The listing builds one solid part. Answer for the finished solid, in the listing's coordinates (mm). Face numbers are marked on the shaded views. A direction names the side the tool comes from. Give positions to 0.01 mm unless a question says otherwise; leave off trailing zeros. Write each loop counter-clockwise with the first axis right and the second up, starting at its lowest first coordinate (ties: lowest second). Pieces come first, ordered by that corner, then holes. Notation, with made-up numbers: (58, 22.25) -> (73, 22.25) arc R26 ccw to (73, 40.25) -> close; hole circle Ø8 at (-31, 70.25). An arc over 180 degrees is marked (long way). Put each result on its own line as item: value. Start each with the question number.
1) A cutting plane is placed at A-A (z = 0). Write down the section's boundary in (x, y), then the cut area to 4 significant figures.
2) For the marked faces 4 and 5, determine the directions among +Z, -Z, +X, -X, +Y, -Y from which every point of the face is accessible in a straight line to the end or side of a thin tool.
3) A cutting plane is placed at D-D (x = 2). Write down the section's boundary in (y, z), then the cut area to 3 significant figures.
4) Flat-ended cylindrical pins translate along their axes: pin 1 Ø1 at (x, z) = (1, 0.5) entering from +Y; pin 2 Ø2 at (x, z) = (-1, -1) entering from +Y. Find the tip coordinate at first contact, or state that the pin passes through.
5) A cutting plane is placed at B-B (x = 0). Write down the section's boundary in (y, z).
6) Find the intervals of material crossed by line 1 along X through (y, z) = (3, 0); line 2 along X through (y, z) = (7.2, 0), in increasing order. Write a range as from..to.
7) A cutting plane is placed at C-C (y = 5). Write down the section's boundary in (x, z).
8) For a pull along X with two mould halves and no side action, classify the marked faces 1, 2 and 3 as released by +X, released by -X, zero draft, split by the parting line, or undercut.
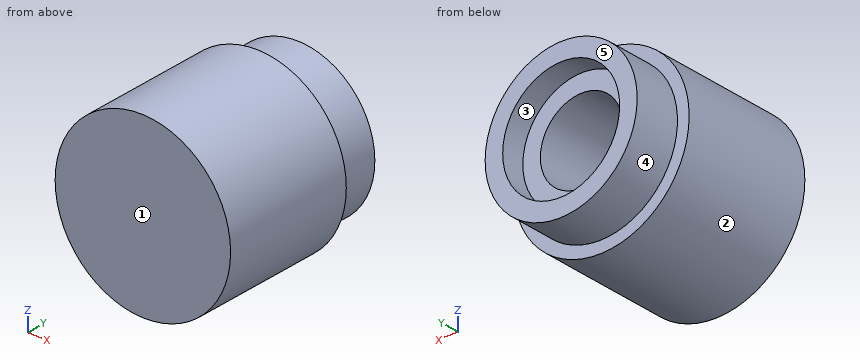
from build123d import *

# Parameters (mm, degrees)
SKETCH1_R           = 3.75
BOSS_EXTRUDE1_DEPTH = 7.75
SKETCH3_R           = 3.75
SKETCH3_R_2         = 3.25
CUT_EXTRUDE1_DEPTH  = 2
SKETCH4_R           = 1.75
CUT_EXTRUDE2_DEPTH  = 7.25
SKETCH5_R           = 2.5
CUT_EXTRUDE3_DEPTH  = 1


with BuildPart() as part:
    # Sketch1 → Boss-Extrude1 (new body)
    with BuildSketch(Plane(origin=(0, 0, 0), x_dir=(1, 0, 0), z_dir=(0, 1, 0))):
        Circle(SKETCH1_R)
    extrude(amount=BOSS_EXTRUDE1_DEPTH)

    # Sketch3 → Cut-Extrude1 (cut)
    with BuildSketch(Plane(origin=(0, 7.75, 0), x_dir=(1, 0, 0), z_dir=(0, 1, 0))):
        Circle(SKETCH3_R)
        Circle(SKETCH3_R_2, mode=Mode.SUBTRACT)
    extrude(amount=-CUT_EXTRUDE1_DEPTH, mode=Mode.SUBTRACT)

    # Sketch4 → Cut-Extrude2 (cut)
    with BuildSketch(Plane(origin=(0, 7.75, 0), x_dir=(1, 0, 0), z_dir=(0, 1, 0))):
        Circle(SKETCH4_R)
    extrude(amount=-CUT_EXTRUDE2_DEPTH, mode=Mode.SUBTRACT)

    # Sketch5 → Cut-Extrude3 (cut)
    with BuildSketch(Plane(origin=(0, 7.75, 0), x_dir=(1, 0, 0), z_dir=(0, 1, 0))):
        Circle(SKETCH5_R)
    extrude(amount=-CUT_EXTRUDE3_DEPTH, mode=Mode.SUBTRACT)


solid = part.part
Reply:
1. outline: (-3.75, 0) -> (3.75, 0) -> (3.75, 5.75) -> (3.25, 5.75) -> (3.25, 7.75) -> (2.5, 7.75) -> (2.5, 6.75) -> (1.75, 6.75) -> (1.75, 0.5) -> (-1.75, 0.5) -> (-1.75, 6.75) -> (-2.5, 6.75) -> (-2.5, 7.75) -> (-3.25, 7.75) -> (-3.25, 5.75) -> (-3.75, 5.75) -> close
1. area: 29.25 mm2
2. face 4: +Y
2. face 5: +Z, -Z, +X, -X, +Y
3. outline: (0, -3.17) -> (5.75, -3.17) -> (5.75, -2.56) -> (7.75, -2.56) -> (7.75, -1.5) -> (6.75, -1.5) -> (6.75, 1.5) -> (7.75, 1.5) -> (7.75, 2.56) -> (5.75, 2.56) -> (5.75, 3.17) -> (0, 3.17) -> close
3. area: 43.7 mm2
4. pin 1: stops at y = 0.5
4. pin 2: stops at y = 6.75
5. outline: (0, -3.75) -> (5.75, -3.75) -> (5.75, -3.25) -> (7.75, -3.25) -> (7.75, -2.5) -> (6.75, -2.5) -> (6.75, -1.75) -> (0.5, -1.75) -> (0.5, 1.75) -> (6.75, 1.75) -> (6.75, 2.5) -> (7.75, 2.5) -> (7.75, 3.25) -> (5.75, 3.25) -> (5.75, 3.75) -> (0, 3.75) -> close
6. line 1: x = -3.75..-1.75, 1.75..3.75
6. line 2: x = -3.25..-2.5, 2.5..3.25
7. outline: circle Ø7.5 at (0, 0); hole circle Ø3.5 at (0, 0)
8. face 1: zero draft
8. face 2: split by the parting line
8. face 3: undercut
